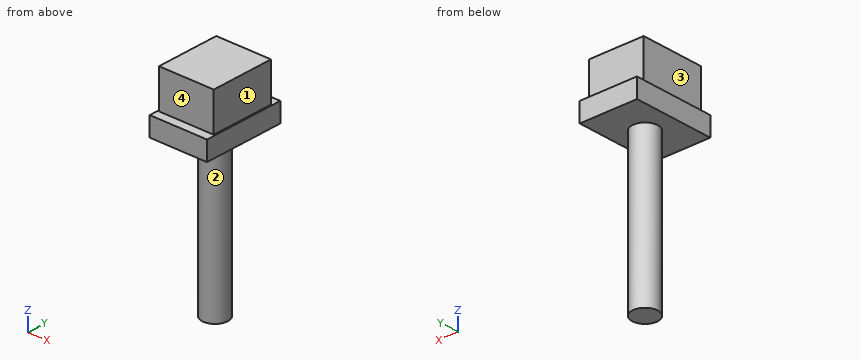
from build123d import *

# Parameters (mm, degrees)
SKETCH038_W  = 4.3
SKETCH038_H  = 5
PAD018_DEPTH = 4.5
SKETCH039_W  = 4.5
SKETCH039_H  = 6.4
PAD019_DEPTH = 1.5
SKETCH040_R  = 1
PAD020_DEPTH = 12.3


with BuildPart() as part:
    # Sketch038 → Pad018 (new body)
    with BuildSketch(Plane.XY):
        with Locations((23.95, 1.9814)):
            Rectangle(SKETCH038_W, SKETCH038_H)
    extrude(amount=PAD018_DEPTH)

    # Sketch039 → Pad019 (join)
    with BuildSketch(Plane.XY):
        with Locations((23.95, 1.9814)):
            Rectangle(SKETCH039_W, SKETCH039_H)
    extrude(amount=PAD019_DEPTH)

    # Sketch040 → Pad020 (join)
    with BuildSketch(Plane.XY):
        with Locations((23.95, 1.98)):
            Circle(SKETCH040_R)
    extrude(amount=-PAD020_DEPTH)


with BuildPart() as part_1:
    # Body005 placement: moved
    add(part.part.moved(Location((0, 0, 6))))


solid = part_1.part
For this review, take the finished solid that the model builds, in its own axes (mm). Face numbers are marked on the shaded views. A direction names the side the tool comes from. Give positions to 0.01 mm unless a question says otherwise; leave off trailing zeros. Loops run counter-clockwise (first coordinate to the right, second up) from the corner with the lowest first, then second, coordinate; pieces in that order, holes last. Notation, with made-up numbers: M 9,-28 L 50,-28 A10 cw 50,-19 Z; hole C 41.25,6 d9. An arc over 180 degrees is marked long. Put each result on its own line as item: value. Start each with the question number.
(1) Add section B-B, the plane y = 1.98. Write out the cut boundary in (x, z).
(2) Add section A-A, the plane x = 23.95. Write out the cut boundary in (y, z).
(3) Add section C-C, the plane z = 0.25. Write out the cut boundary in (x, y), then the cut area to 3 significant figures.
(4) Add section D-D, the plane x = 22.15. Write out the cut boundary in (y, z).
(5) Wall thickness on L1, parallel to Z at x = 23.9, y = 4; L2, parallel to Y at x = 22.55, z = 9.75; L3, parallel to Z at x = 23.7, y = -1: over which ranges is each line inside the solid? List them lowest first.
(6) For pin 1 (3.5 mm diameter, centred on y = 1.5, z = 9, fed in from +X); pin 2 (0.9 mm diameter, centred on x = 23, z = 9.5, fed in from -Y); pin 3 (2.5 mm diameter, centred on y = 2, z = 9, fed in from -X); pin 4 (3 mm diameter, centred on y = 0, z = 0, fed in from -X), all flat-tipped, find the tip position at first contact; note any pin that passes through.
(7) Machinability: for the marked faces 1, 2, 3 and 4, which of the approach directions +Z, -Z, +X, -X, +Y, -Y give a long, thin tool a straight path to every point of the face, cutting with its end or side? Answer none if there is none.
Result:
1. outline: M 21.7,6 L 22.95,6 L 22.95,-6.3 L 24.95,-6.3 L 24.95,6 L 26.2,6 L 26.2,7.5 L 26.1,7.5 L 26.1,10.5 L 21.8,10.5 L 21.8,7.5 L 21.7,7.5 Z
2. outline: M -1.22,6 L 0.98,6 L 0.98,-6.3 L 2.98,-6.3 L 2.98,6 L 5.18,6 L 5.18,7.5 L 4.48,7.5 L 4.48,10.5 L -0.52,10.5 L -0.52,7.5 L -1.22,7.5 Z
3. outline: C 23.95,1.98 d2
3. area: 3.14 mm^2
4. outline: M -1.22,6 L 5.18,6 L 5.18,7.5 L 4.48,7.5 L 4.48,10.5 L -0.52,10.5 L -0.52,7.5 L -1.22,7.5 Z
5. L1: z = 6 to 10.5
5. L2: y = -0.52 to 4.48
5. L3: z = 6 to 7.5
6. pin 1: stops at x = 26.2
6. pin 2: stops at y = -0.52
6. pin 3: stops at x = 21.8
6. pin 4: stops at x = 23.07
7. face 1: +Z, +X, +Y, -Y
7. face 2: -Z
7. face 3: +Z, -X, +Y, -Y
7. face 4: +Z, +X, -X, -Y
